The figure shows three views and two pictorial views of one solid part (mm, origin at its lowest corner). Answer the questions. A direction names the side the tool comes from. Coordinates: 2 decimals unless noted, no trailing zeros. Loops run counter-clockwise (first coordinate to the right, second up) from the corner with the lowest first, then second, coordinate; pieces in that order, holes last. Notation, with made-up numbers: (33.25, 19.5) -> (47.25, 19.5) arc R16 cw to (47.25, 35.5) -> close; hole circle Ø11 at (-30, 89.5). An arc over 180 degrees is marked (long way). Use a Markdown table: item, result. Add a question column.
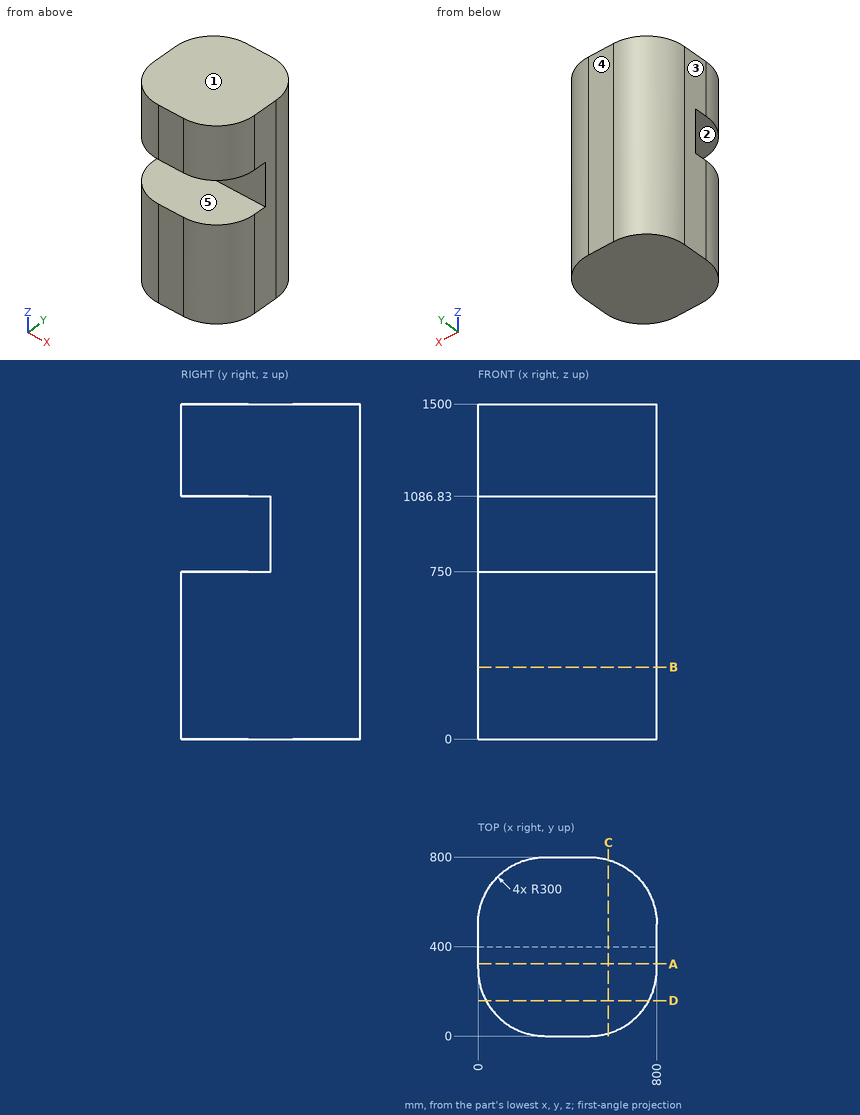
Item 1: Given pin 1 (12 mm diameter, centred on x = 151, z = 775.5, fed in from -Y); pin 2 (8 mm diameter, centred on y = 566.5, z = 1248, fed in from +X); pin 3 (12 mm diameter, centred on x = 113, z = 649, fed in from +Y), each flat-ended and moving along its own axis, determine where each tip first touches the part or whether it passes through.
Item 2: Find the intervals of material crossed by probe 1 along Z at (x, y) = (180.5, 338); probe 2 along Y at (x, z) = (401.5, 895.5); probe 3 along X at (y, z) = (248, 1340), in increasing order.
Item 3: For a pull along Z with two mould halves and no side action, classify the marked faces 1, 2 and 3 as +Z half, -Z half, draft (parallel to the pull), parting line (faces both ways), or undercut.
Item 4: Section B-B (z = 322.5) is taken. Determine the outline of the cut face in (x, y).
Item 5: Section C-C (x = 583) is taken. Determine the outline of the cut face in (y, z), then the cut area to 3 significant figures.
Item 6: For the marked faces 4 and 5, determine the directions among +Z, -Z, +X, -X, +Y, -Y from which every point of the face is accessible in a straight line to the end or side of a thin tool.
Item 7: Section A-A (y = 322.5) is taken. Determine the outline of the cut face in (x, z).
Item 8: Section D-D (y = 158) is taken. Determine the outline of the cut face in (x, z) (1 decimal), then the cut area to 3 significant figures.
Output:
| question | item | result |
|---|---|---|
| 1 | pin 1 | stops at y = 400 |
| 1 | pin 2 | stops at x = 793.42 |
| 1 | pin 3 | stops at y = 739.25 |
| 2 | probe 1 | z = 0 to 750, 1086.83 to 1500 |
| 2 | probe 2 | y = 400 to 800 |
| 2 | probe 3 | x = 4.54 to 795.46 |
| 3 | face 1 | +Z half |
| 3 | face 2 | undercut |
| 3 | face 3 | draft |
| 4 | outline | (0, 300) arc R300 ccw to (300, 0) -> (500, 0) arc R300 ccw to (800, 300) -> (800, 500) arc R300 ccw to (500, 800) -> (300, 800) arc R300 ccw to (0, 500) -> close |
| 5 | outline | (11.71, 0) -> (788.29, 0) -> (788.29, 1500) -> (11.71, 1500) -> (11.71, 1086.83) -> (400, 1086.83) -> (400, 750) -> (11.71, 750) -> close |
| 5 | area | 1,030,000 mm2 |
| 6 | face 4 | +Z, -Z, +X, -X, +Y |
| 6 | face 5 | +X, -X, -Y |
| 7 | outline | (0, 0) -> (800, 0) -> (800, 750) -> (0, 750) -> close; (0, 1086.83) -> (800, 1086.83) -> (800, 1500) -> (0, 1500) -> close |
| 8 | outline | (35.7, 0) -> (764.3, 0) -> (764.3, 750) -> (35.7, 750) -> close; (35.7, 1086.8) -> (764.3, 1086.8) -> (764.3, 1500) -> (35.7, 1500) -> close |
| 8 | area | 847,000 mm2 |
